from build123d import *

# Parameters (mm, degrees)
SM_BASE_FLANGE_1_DEPTH           = 410
CUT_EXTRUDE_1_DEPTH              = 438.623696799
SM_EDGE_FLANGE_1_STRIP_W         = 9
SM_EDGE_FLANGE_1_STRIP_H         = 1.5
SM_EDGE_FLANGE_1_STRIP_CUT_DEPTH = 118
SM_EDGE_FLANGE_1_DEPTH           = 118


# Sheet-metal steps are written as plain solids
with BuildPart() as part:
    # Sketch 1 → Базовая кромка1 (new body)
    with BuildSketch(Plane(origin=(0, 0, 0), x_dir=(0, 0, -1), z_dir=(1, 0, 0))):
        with BuildLine():
            Line((0, 0), (-148.5, 0))
            ThreePointArc((-148.5, 0), (-149.560660172, -0.439339828), (-150, -1.5))
            Line((-150, -1.5), (-150, -20))
            Line((-150, -20), (-151.5, -20))
            Line((-151.5, -20), (-151.5, -1.5))
            ThreePointArc((-151.5, -1.5), (-150.621320344, 0.621320344), (-148.5, 1.5))
            Line((-148.5, 1.5), (0, 1.5))
            Line((0, 1.5), (0, 0))
        make_face()
    extrude(amount=-SM_BASE_FLANGE_1_DEPTH)

    # Эскиз9 → Вырез-Вытянуть1 (cut, through all)
    with BuildSketch(Plane(origin=(0, 1.5, 0), x_dir=(1, 0, 0), z_dir=(0, 1, 0))):
        with BuildLine():
            Line((-410, -118), (-400, -118))
            ThreePointArc((-400, -118), (-398.585786438, -118.585786438), (-398, -120))
            Line((-398, -120), (-398, -151.5))
            Line((-398, -151.5), (-410, -151.5))
            Line((-410, -151.5), (-410, -118))
        make_face()
    extrude(amount=-CUT_EXTRUDE_1_DEPTH, mode=Mode.SUBTRACT)

    # Ребро-кромка1 strip (across the edge) → Ребро-кромка1 strip cut (cut)
    with BuildSketch(Plane(origin=(-410, 0, 118), x_dir=(1, 0, 0), z_dir=(0, 0, -1))):
        with Locations((-3, -0.75)):
            Rectangle(SM_EDGE_FLANGE_1_STRIP_W, SM_EDGE_FLANGE_1_STRIP_H)
    extrude(amount=SM_EDGE_FLANGE_1_STRIP_CUT_DEPTH, mode=Mode.SUBTRACT)

    # Ребро-кромка1 section (across the edge) → Ребро-кромка1 (add)
    with BuildSketch(Plane(origin=(-410, 0, 118), x_dir=(1, 0, 0), z_dir=(0, 0, -1))):
        with BuildLine():
            Line((-1.5, 1.5), (-1.5, 20))
            Line((-1.5, 20), (0, 20))
            Line((0, 20), (0, 1.5))
            ThreePointArc((0, 1.5), (0.439339828, 0.439339828), (1.5, 0))
            Line((1.5, 0), (1.5, -1.5))
            ThreePointArc((1.5, -1.5), (-0.621320344, -0.621320344), (-1.5, 1.5))
        make_face()
    extrude(amount=SM_EDGE_FLANGE_1_DEPTH)

    # Зеркальное отражение1: part across plane


with BuildPart() as part_1:
    add(part.part)
    add(part.part.mirror(Plane(origin=(-568.017972801, 1.5, 0), x_dir=(1, 0, 0), z_dir=(0, 0, 1))))

    # Зеркальное отражение2: part across plane


with BuildPart() as part_2:
    add(part_1.part)
    add(part_1.part.mirror(Plane(origin=(0, 1.5, 148.5), x_dir=(0, 0, 1), z_dir=(1, 0, 0))))


solid = part_2.part
For this review, take the finished solid that the model builds, in its own axes (mm). A direction names the side the tool comes from. Coordinates: 2 decimals unless noted, no trailing zeros. Loops run counter-clockwise (first coordinate to the right, second up) from the corner with the lowest first, then second, coordinate; pieces in that order, holes last. Notation, with made-up numbers: (-27, -35.5) - (-10, -35.5) arc R22 ccw to (-10, -8.5) - close; hole circle Ø5 at (46, 81). An arc over 180 degrees is marked (long way). Use a Markdown table: item, result. Add a question column.
Item 1: Insertion check: pin 1 Ø6 at (x, y) = (-403, -9.5) entering from +Z. The pin has a flat end and moves straight along its axis. Give the tip position at first contact, or say it passes through.
Item 2: We need section A-A (y = -7.75). Give the boundary of the cut face in (x, z), and give its area (3 significant figures).
Item 3: For line 1 (Z direction, x = -270, y = -15.5); line 2 (X direction, y = -6.5, z = 81.5); line 3 (Y direction, x = 124, z = 65), list the stretches that pass through material, from the lowest coordinate up.
Item 4: We need section B-B (z = -87.5). Give the boundary of the cut face in (x, y).
Item 5: Tool access review of faces 4 (the face through (398, 0.4, -140.3)), 5 (the face through (410, -11, -2)), 6 (the face through (-6, -11, -150)), 7 (the face through (-398, 0.4, -140.3)): name each direction out of +Z, -Z, +X, -X, +Y, -Y from which nothing blocks a thin tool from reaching the whole face with its end or side.
Item 6: We need section C-C (x = 200). Give the boundary of the cut face in (y, z), and give its area (3 significant figures).
Item 7: Mouldability with a two-part tool opening along X and no side actions: class faces 1 (the face through (-6, -11, 150)), 2 (the face through (-6, 0, 2)), 3 (the face through (-398, 0.4, 140.3)) as pulls with the +X half, pulls with the -X half, needs draft (parallel to the pull), parting line crosses it, or undercut.
Results list:
| question | item | result |
|---|---|---|
| 1 | pin 1 | passes through |
| 2 | outline | (-411.5, -118) - (-410, -118) - (-410, 118) - (-411.5, 118) - close; (-398, -151.5) - (398, -151.5) - (398, -150) - (-398, -150) - close; (-398, 150) - (398, 150) - (398, 151.5) - (-398, 151.5) - close; (410, -118) - (411.5, -118) - (411.5, 118) - (410, 118) - close |
| 2 | area | 3,100 mm^2 |
| 3 | line 1 | z = -151.5 to -150, 150 to 151.5 |
| 3 | line 2 | x = -411.5 to -410, 410 to 411.5 |
| 3 | line 3 | y = 0 to 1.5 |
| 4 | outline | (-411.5, -20) - (-410, -20) - (-410, -1.5) arc R1.5 cw to (-408.5, 0) - (408.5, 0) arc R1.5 cw to (410, -1.5) - (410, -20) - (411.5, -20) - (411.5, -1.5) arc R3 ccw to (408.5, 1.5) - (-408.5, 1.5) arc R3 ccw to (-411.5, -1.5) - close |
| 5 | face 4 | -Z, +X, +Y, -Y |
| 5 | face 5 | +Z, -Z, -Y |
| 5 | face 6 | +X, -X, -Y |
| 5 | face 7 | -Z, -X, +Y, -Y |
| 6 | outline | (-20, -151.5) - (-1.5, -151.5) arc R3 ccw to (1.5, -148.5) - (1.5, 148.5) arc R3 ccw to (-1.5, 151.5) - (-20, 151.5) - (-20, 150) - (-1.5, 150) arc R1.5 cw to (0, 148.5) - (0, -148.5) arc R1.5 cw to (-1.5, -150) - (-20, -150) - close |
| 6 | area | 512 mm^2 |
| 7 | face 1 | needs draft |
| 7 | face 2 | undercut |
| 7 | face 3 | pulls with the -X half |
